The listing builds one solid part. Answer for the finished solid, in the listing's coordinates (mm). Face numbers are marked on the shaded views. A direction names the side the tool comes from. Coordinates: 2 decimals unless noted, no trailing zeros. Loops run counter-clockwise (first coordinate to the right, second up) from the corner with the lowest first, then second, coordinate; pieces in that order, holes last. Notation, with made-up numbers: M 47,-2.5 L 73,-2.5 A34 cw 73,27.5 Z; hole C 45.5,14 d3. An arc over 180 degrees is marked long. Return JSON: item names as keys, results as strings. Group by question number.
1. Section B-B (x = -27.5) is taken. Write down the section's boundary in (y, z), then the cut area to 4 significant figures.
2. Straight lines are drawn through the part: L1, parallel to X at y = 3.5, z = 36.5; L2, parallel to Y at x = -36.5, z = -33; L3, parallel to Z at x = -40, y = 23.5. For each, find the intervals that lie inside material, in ascending order. Write a range as from..to.
3. Section A-A (y = 22) is taken. Write down the section's boundary in (x, z), then the cut area to 4 significant figures.
4. Section D-D (z = -3) is taken. Write down the section's boundary in (x, y).
5. Section C-C (z = -31.5) is taken. Write down the section's boundary in (x, y), then the cut area to 4 significant figures.
6. Which of the six approach directions +Z, -Z, +X, -X, +Y, -Y give full straight-line access (tool end or side, diameter ignored) to the marked faces 1, 2 and 3?
7. Given P1, Ø1, axis at x = -21.5, y = 15, coming from the +Z side; P2, Ø6, axis at y = 22.5, z = 38.5, coming from the -X side; P3, Ø10.5, axis at y = 17, z = 2.5, coming from the +X side, each flat-ended and moving along its own axis, determine where each tip first touches the part or whether it passes through.
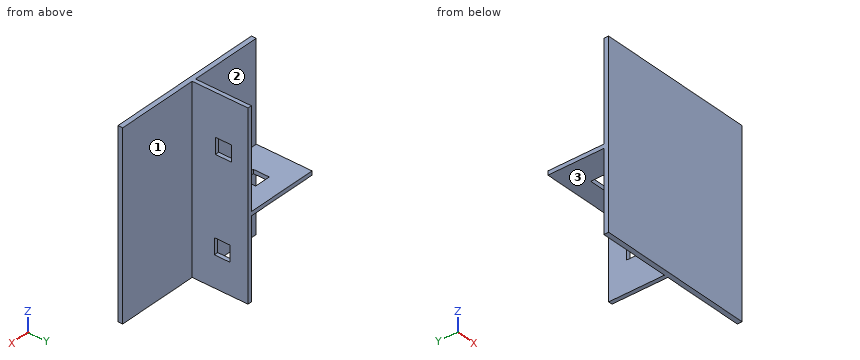
```python
from build123d import *

# Parameters (mm, degrees)
SKETCH1_W           = 99
SKETCH1_H           = 114
BOSS_EXTRUDE1_DEPTH = 3
BOSS_EXTRUDE2_DEPTH = 35
SKETCH3_W           = 10
SKETCH3_H           = 10
CUT_EXTRUDE1_DEPTH  = 35
SKETCH4_W           = 10
SKETCH4_H           = 10
CUT_EXTRUDE2_DEPTH  = 35


with BuildPart() as part:
    # Sketch1 → Boss-Extrude1 (new body)
    with BuildSketch(Plane(origin=(0, 0, 0), x_dir=(1, 0, 0), z_dir=(0, 1, 0))):
        Rectangle(SKETCH1_W, SKETCH1_H)
    extrude(amount=BOSS_EXTRUDE1_DEPTH)

    # Sketch2 → Boss-Extrude2 (add)
    with BuildSketch(Plane(origin=(0, 3, 0), x_dir=(1, 0, 0), z_dir=(0, 1, 0))):
        Polygon((-2, 57), (-4.5, 57), (-4.5, 7), (-49.5, 7), (-49.5, 4.5), (-4.5, 4.5), (-4.5, -57), (-2, -57), align=None)
    extrude(amount=BOSS_EXTRUDE2_DEPTH)

    # Sketch3 → Cut-Extrude1 (cut)
    with BuildSketch(Plane.XY.offset(-4.5)):
        with Locations((-27.352089656, 20.663342565)):
            Rectangle(SKETCH3_W, SKETCH3_H)
    extrude(amount=-CUT_EXTRUDE1_DEPTH, mode=Mode.SUBTRACT)

    # Sketch4 → Cut-Extrude2 (cut)
    with BuildSketch(Plane.ZY.offset(4.5)):
        with Locations((-32.678506246, 21.863269453)):
            Rectangle(SKETCH4_W, SKETCH4_H)
        with Locations((25.912956103, 22.537357248)):
            Rectangle(SKETCH4_W, SKETCH4_H)
    extrude(amount=-CUT_EXTRUDE2_DEPTH, mode=Mode.SUBTRACT)


solid = part.part
```
Worked out:
{
 "1": {"outline": "M 0,-57 L 3,-57 L 3,-7 L 15.66,-7 L 15.66,-4.5 L 3,-4.5 L 3,57 L 0,57 Z; M 25.66,-7 L 38,-7 L 38,-4.5 L 25.66,-4.5 Z", "area": "404.5 mm^2"},
 "2": {"L1": "-4.5..-2", "L2": "0..3", "L3": "-7..-4.5"},
 "3": {"outline": "M -49.5,-7 L -32.35,-7 L -32.35,-4.5 L -49.5,-4.5 Z; M -22.35,-7 L -4.5,-7 L -4.5,-27.68 L -2,-27.68 L -2,20.91 L -4.5,20.91 L -4.5,-4.5 L -22.35,-4.5 Z; M -4.5,-57 L -2,-57 L -2,-37.68 L -4.5,-37.68 Z; M -4.5,30.91 L -2,30.91 L -2,57 L -4.5,57 Z", "area": "322.5 mm^2"},
 "4": {"outline": "M -49.5,0 L 49.5,0 L 49.5,3 L -2,3 L -2,38 L -4.5,38 L -4.5,3 L -49.5,3 Z"},
 "5": {"outline": "M -49.5,0 L 49.5,0 L 49.5,3 L -2,3 L -2,16.86 L -4.5,16.86 L -4.5,3 L -49.5,3 Z; M -4.5,26.86 L -2,26.86 L -2,38 L -4.5,38 Z", "area": "359.5 mm^2"},
 "6": {"face 1": "+Z, -Z, +X, +Y", "face 2": "+Z, -X, +Y", "face 3": "-Z, -X, +Y"},
 "7": {"P1": "z = -4.5", "P2": "x = -4.5", "P3": "x = -2"}
}
